Source: CAD feature listing. Evaluate the final solid. Frame: model axes, mm. Round coordinates to 2 decimals unless told otherwise and drop trailing zeros. Order: outer loops, then holes, each group sorted by start corner. A loop starts at its lowest first (then second) coordinate and runs counter-clockwise, first axis right, second up. Notation, with made-up numbers: (-20.75, 10.25) - (20.25, 10.25) arc R14 ccw to (20.25, 18.25) - close; hole circle Ø9 at (84, 56). An arc over 180 degrees is marked (long way). Put each result on its own line as item: value. Start each with the question number.
1) Line query: probe 1 along X at (y, z) = (139.5, 115); probe 2 along Z at (x, y) = (317.5, 148); probe 3 along Z at (x, y) = (291, 14). Output: solid intervals per line, ascending. Write a range as [from, to].
2) Contact query for flat-ended pins moving along their axis: P1, Ø12, axis at y = -40.5, z = 376, coming from the +X side; P2, Ø13.5, axis at x = 313, z = 713, coming from the +Y side; P3, Ø12.5, axis at y = -38.5, z = 807, coming from the +X side; P4, Ø15, axis at x = 308, y = 71.5, coming from the -Z side. Output: stop coordinate, or through.
3) Section B-B on z = 283.5. Output: boundary loops of the cut face in (x, y), then the cut area to 3 significant figures.
4) Section A-A on y = -30. Output: boundary loops of the cut face in (x, z), then the cut area to 3 significant figures.
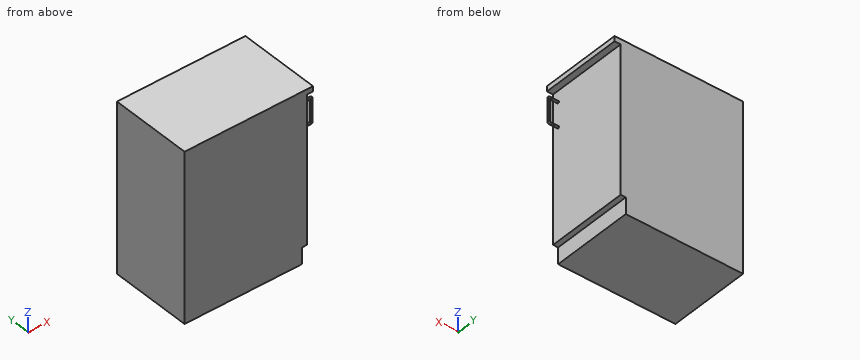
```python
from build123d import *

# Parameters (mm, degrees)
F0_W        = 600
F0_H        = 400
F1_DEPTH    = 800
F2_W        = 400
F2_H        = 80
F3_DEPTH    = 25
F5_DEPTH    = 50
F6_T1_DEPTH = 120
F6_T4_ANGLE = 180
F6_T6_ANGLE = 180
F7_W        = 40
F7_H        = 110
F8_DEPTH    = 25
F9_R        = 4.99999
F10_W       = 630
F10_H       = 400
F11_DEPTH   = 25


# Not quite as in the source:
# - a fillet or chamfer that OpenCascade refuses, or shapes differently, is made with other operations: its cross-section is extruded or revolved along the edge and cut away or added
# - a fillet or chamfer is up to 0.001 mm smaller than in the source, because OpenCascade refuses the exact size


with BuildPart() as f1:
    # F0 (on Top) → F1 (new body)
    with BuildSketch(Plane.XY):
        Rectangle(F0_W, F0_H)
    extrude(amount=F1_DEPTH)

    # F2 (on face) → F3 (cut)
    with BuildSketch(Plane.YZ.offset(300)):
        with Locations((0, 40)):
            Rectangle(F2_W, F2_H)
    extrude(amount=-F3_DEPTH, mode=Mode.SUBTRACT)

    # F4 (on face) → F5 (join)
    with BuildSketch(Plane.YZ.offset(300)):
        with BuildLine():
            ThreePointArc((-170, 750), (-173.5355339059, 748.5355339059), (-175, 745))
            Line((-175, 745), (-175, 625))
            ThreePointArc((-175, 625), (-173.5355339059, 621.4644660941), (-170, 620))
            ThreePointArc((-170, 620), (-166.4644660941, 621.4644660941), (-165, 625))
            Line((-165, 625), (-165, 745))
            ThreePointArc((-165, 745), (-166.4644660941, 748.5355339059), (-170, 750))
        make_face()
    extrude(amount=F5_DEPTH)

    # F6: fillet of radius 5 on 4 edges, made by hand

    # F6_s2 → F6_t1 (cut)
    with BuildSketch(Plane.XY.offset(625)):
        with BuildLine():
            ThreePointArc((345, -175), (348.5355339059, -173.5355339059), (350, -170))
            Line((350, -170), (350, -175))
            Line((350, -175), (345, -175))
        make_face()
        with BuildLine():
            ThreePointArc((345, -165), (348.5355339059, -166.4644660941), (350, -170))
            Line((350, -170), (350, -165))
            Line((350, -165), (345, -165))
        make_face()
    extrude(amount=F6_T1_DEPTH, mode=Mode.SUBTRACT)

    # F6_s3 → F6_t4 (revolve, cut)
    with BuildSketch(Plane.XY.offset(745)):
        with BuildLine():
            ThreePointArc((345, -175), (348.5355339059, -173.5355339059), (350, -170))
            Line((350, -170), (350, -175))
            Line((350, -175), (345, -175))
        make_face()
    revolve(axis=Axis((350, -170, 745), (-1, 0, 0)), revolution_arc=F6_T4_ANGLE, mode=Mode.SUBTRACT)

    # F6_s5 → F6_t6 (revolve, cut)
    with BuildSketch(Plane.XY.offset(625)):
        with BuildLine():
            ThreePointArc((345, -165), (348.5355339059, -166.4644660941), (350, -170))
            Line((350, -170), (350, -165))
            Line((350, -165), (345, -165))
        make_face()
    revolve(axis=Axis((350, -170, 625), (-1, 0, 0)), revolution_arc=F6_T6_ANGLE, mode=Mode.SUBTRACT)

    # F7 (on face) → F8 (cut)
    with BuildSketch(Plane(origin=(0, -165, 0), x_dir=(-1, 0, 0), z_dir=(0, 1, 0))):
        with Locations((-320, 685)):
            Rectangle(F7_W, F7_H)
    extrude(amount=-F8_DEPTH, mode=Mode.SUBTRACT)

    # F9 (radius 5 in the source; OpenCascade refuses exactly that, so slightly less here)
    f9_edges = [f1.edges().sort_by_distance(p)[0] for p in [
        (320, -165, 740),
        (340, -165, 685),
        (320, -165, 630),
        (320, -175, 740),
        (340, -175, 685),
        (320, -175, 630),
    ]]
    fillet(f9_edges, radius=F9_R)

    # F10 (on face) → F11 (join)
    with BuildSketch(Plane.XY.offset(800)):
        with Locations((15, 0)):
            Rectangle(F10_W, F10_H)
    extrude(amount=F11_DEPTH)


solid = f1.part
```
Answer sheet:
1. probe 1: [-300, 300]
1. probe 2: [800, 825]
1. probe 3: [80, 825]
2. P1: x = 300
2. P2: through
2. P3: x = 330
2. P4: z = 800
3. outline: (-300, -200) - (300, -200) - (300, 200) - (-300, 200) - close
3. area: 240,000 mm^2
4. outline: (-300, 0) - (275, 0) - (275, 80) - (300, 80) - (300, 800) - (330, 800) - (330, 825) - (-300, 825) - close
4. area: 494,000 mm^2
